Read the model definition and answer for the solid it produces. Units are mm, in the model's axes. A direction names the side the tool comes from. Give positions to 0.01 mm unless a question says otherwise; leave off trailing zeros. Order: outer loops, then holes, each group sorted by start corner. A loop starts at its lowest first (then second) coordinate and runs counter-clockwise, first axis right, second up.
Item 1: The mould has two halves that part along Y. Classify faces 5 (the face through (13, -25.4, 3)), 6 (the face through (9.525, -13, 3)), 7 (the face through (19.05, -5, 14)): +Y half, -Y half, draft (parallel to the pull), parting line (faces both ways), or undercut.
Item 2: A cutting plane is placed at C-C (z = 4.5). Write down the section's boundary in (x, y) (3 decimals), plus the area to 3 significant figures.
Item 3: Given pin 1 Ø4 at (x, z) = (32, 7) entering from -Y; pin 2 Ø3 at (y, z) = (-16.5, 3.5) entering from +X; pin 3 Ø6 at (x, y) = (17.5, -20) entering from +Z; pin 4 Ø2 at (x, y) = (32, -15) entering from +Z, each flat-ended and moving along its own axis, determine where each tip first touches the part or whether it passes through.
Item 4: A cutting plane is placed at A-A (z = 22). Write down the section's boundary in (x, y), plus the area to 3 significant figures.
Item 5: Find the intervals of material crossed by line 1 along X through (y, z) = (-11.25, 13.25); line 2 along Y through (x, z) = (20.5, 1.5), in increasing order.
Item 6: A cutting plane is placed at D-D (y = -2.5). Write down the section's boundary in (x, z), plus the area to 3 significant figures.
Item 7: Which of the six approach directions +Z, -Z, +X, -X, +Y, -Y give full straight-line access (tool end or side, diameter ignored) to faces 1 (the face through (6.35, -7, 14)), 2 (the face through (19.05, -19, 3)), 3 (the face through (6.35, -24, 5)), 4 (the face through (15.875, -13, 3))?
Item 8: A cutting plane is placed at B-B (y = -13.75). Write down the section's boundary in (x, z) (3 decimals), plus the area to 3 significant figures.
from build123d import *

# Parameters (mm, degrees)
F1_DEPTH = 25.4
F2_W     = 12.7
F2_H     = 25.4
F3_DEPTH = 19.05
F5_DEPTH = 19.05
F7_DEPTH = 6.35
F9_DEPTH = 25.4


with BuildPart() as f1:
    # F0 (on Front) → F1 (new body)
    with BuildSketch(Plane.XZ):
        Polygon((0, 25.4), (0, 0), (38.1, 0), (38.1, 25.4), (19.05, 25.4), (19.05, 6.35), (6.35, 6.35), (6.35, 25.4), align=None)
    extrude(amount=F1_DEPTH)

    # F2 (on face) → F3 (cut)
    with BuildSketch(Plane.YZ.offset(38.1)):
        with Locations((-19.05, 12.7)):
            Rectangle(F2_W, F2_H)
    extrude(amount=-F3_DEPTH, mode=Mode.SUBTRACT)

    # F4 (on face) → F5 (cut)
    with BuildSketch(Plane.YZ.offset(38.1)):
        Polygon((-12.7, 25.4), (-12.7, 12.7), (0, 25.4), align=None)
    extrude(amount=-F5_DEPTH, mode=Mode.SUBTRACT)

    # F6 (on face) → F7 (cut)
    with BuildSketch(Plane(origin=(0, 0, 0), x_dir=(0, -1, 0), z_dir=(-1, 0, 0))):
        Polygon((25.4, 25.4), (0, 25.4), (25.4, 0), align=None)
    extrude(amount=-F7_DEPTH, mode=Mode.SUBTRACT)

    # F8 (on face) → F9 (cut)
    with BuildSketch(Plane.XY.offset(6.35)):
        with BuildLine():
            ThreePointArc((12.7, -22.225), (14.945064, -21.295064), (15.875, -19.05))
            ThreePointArc((15.875, -19.05), (12.7, -15.875), (9.525, -19.05))
            ThreePointArc((9.525, -19.05), (10.454936, -21.295064), (12.7, -22.225))
        make_face()
        with BuildLine():
            ThreePointArc((9.525, -19.05), (12.7, -15.875), (15.875, -19.05))
            Line((15.875, -19.05), (15.875, -6.35))
            ThreePointArc((15.875, -6.35), (12.7, -9.525), (9.525, -6.35))
            Line((9.525, -6.35), (9.525, -19.05))
        make_face()
        with BuildLine():
            ThreePointArc((9.525, -6.35), (12.7, -9.525), (15.875, -6.35))
            ThreePointArc((15.875, -6.35), (14.945064, -4.104936), (12.7, -3.175))
            ThreePointArc((12.7, -3.175), (10.454936, -4.104936), (9.525, -6.35))
        make_face()
    extrude(amount=-F9_DEPTH, mode=Mode.SUBTRACT)


solid = f1.part
Response values:
1. face 5: -Y half
1. face 6: undercut
1. face 7: draft
2. outline: (0, -20.9) - (6.35, -20.9) - (6.35, -25.4) - (19.05, -25.4) - (19.05, -12.7) - (38.1, -12.7) - (38.1, 0) - (0, 0) - close; hole (9.525, -19.05) arc R3.175 ccw to (15.875, -19.05) - (15.875, -6.35) arc R3.175 ccw to (9.525, -6.35) - close
2. area: 585 mm2
3. pin 1: stops at y = -12.7
3. pin 2: stops at x = 19.05
3. pin 3: stops at z = 6.35
3. pin 4: passes through
4. outline: (0, -3.4) - (6.35, -3.4) - (6.35, 0) - (0, 0) - close; (19.05, -3.4) - (38.1, -3.4) - (38.1, 0) - (19.05, 0) - close
4. area: 86.4 mm2
5. line 1: x = 0 to 6.35, 19.05 to 38.1
5. line 2: y = -12.7 to 0
6. outline: (0, 0) - (38.1, 0) - (38.1, 22.9) - (19.05, 22.9) - (19.05, 6.35) - (6.35, 6.35) - (6.35, 22.9) - (0, 22.9) - close
6. area: 662 mm2
7. face 1: +Z, +Y, -Y
7. face 2: +Z, -Z, +X, -Y
7. face 3: +Z, -X, -Y
7. face 4: +Z, -Z
8. outline: (0, 0) - (9.525, 0) - (9.525, 6.35) - (6.35, 6.35) - (6.35, 11.65) - (0, 11.65) - close; (15.875, 0) - (19.05, 0) - (19.05, 6.35) - (15.875, 6.35) - close
8. area: 114 mm2
